Design review of the part built by this model. Coordinates are the model's own, in mm. Round coordinates to 2 decimals unless told otherwise and drop trailing zeros. Write each loop counter-clockwise with the first axis right and the second up, starting at its lowest first coordinate (ties: lowest second). Pieces come first, ordered by that corner, then holes. Notation, with made-up numbers: (64, 45) -> (84, 45) arc R17 ccw to (84, 49) -> close; hole circle Ø4 at (36, 32.5). An arc over 180 degrees is marked (long way). One line per question, with ' | ' between items. Start each with the question number.
1) Consider section A-A (x = 12). Give the boundary of the cut face in (y, z), then the cut area to 3 significant figures.
2) Consider section C-C (y = -17.5). Give the boundary of the cut face in (x, z), then the cut area to 3 significant figures.
3) Consider section B-B (y = -11.5). Give the boundary of the cut face in (x, z).
4) For probe 1 along Y at (x, z) = (12, 1.45); probe 2 along X at (y, z) = (-31, 5.1); probe 3 along X at (y, z) = (-5.5, 4.85), list the stretches that pass through material, from the lowest coordinate up.
5) Mouldability with a two-part tool opening along Y and no side actions: class faces 1 (the flat face through (90, -18, 3)), 2 (the cylindrical face through (10.4, -22.3, 3)), 3 (the flat face through (46, 0, 3)) as +Y half, -Y half, draft (parallel to the pull), parting line (faces both ways), or undercut.
6) Consider section D-D (z = 1). Count the separate pieces of the cut face and the enclosed holes in it, then the cut area to 3 significant figures.
Autodesk Inventor part; units mm, degrees
ref_plane "YZ Plane" through (0, 0, 0) normal (1, 0, 0) x (0, 1, 0)
ref_plane "XZ Plane" through (0, 0, 0) normal (0, 1, 0) x (-1, 0, 0)
ref_plane "XY Plane" through (0, 0, 0) normal (0, 0, 1) x (1, 0, 0)
sketch "Esboço1" plane through (0, 0, 0) normal (0, 0, 1) x (1, 0, 0)
  line L0 (90, 0) -> (0, 0)
  line L1 (0, 0) -> (0, -35)
  line L2 (0, -35) -> (90, -35)
  line L3 (90, -35) -> (90, 0)
  circle A0 centre (65.3687, -7.1) radius 2.3
  circle A1 centre (23.3687, -29.5996) radius 2.3
  circle A2 centre (44.3687, -27.9) radius 2.3
  circle A3 centre (44.3687, -7.1) radius 2.3
  circle A4 centre (84.63, -17.5) radius 2.3
  circle A5 centre (5.3687, -17.5) radius 2.3
  circle A6 centre (65.3687, -27.9) radius 2.3
  circle A7 centre (23.3687, -5.4004) radius 2.3
  circle A8 centre (12, -11.5) radius 2
  circle A9 centre (12, -23.5) radius 2
  circle A10 centre (76, -17.5) radius 2
  circle A11 centre (6.2932, -5.4004) radius 2.3
  circle A12 centre (6.2932, -29.5996) radius 2.3
  circle A13 centre (82.6841, -5.4004) radius 2.3
  circle A14 centre (82.6768, -29.5996) radius 2.3
extrude "Extrusão1" add sketch "Esboço1" along normal blind 6
properties part number "acrilico frontal" material "Acrílico, transparente"
From the geometry:
1) outline: (-35, 0) -> (-25.5, 0) -> (-25.5, 6) -> (-35, 6) -> close; (-21.5, 0) -> (-13.5, 0) -> (-13.5, 6) -> (-21.5, 6) -> close; (-9.5, 0) -> (0, 0) -> (0, 6) -> (-9.5, 6) -> close | area: 162 mm2
2) outline: (0, 0) -> (3.07, 0) -> (3.07, 6) -> (0, 6) -> close; (7.67, 0) -> (74, 0) -> (74, 6) -> (7.67, 6) -> close; (78, 0) -> (82.33, 0) -> (82.33, 6) -> (78, 6) -> close; (86.93, 0) -> (90, 0) -> (90, 6) -> (86.93, 6) -> close | area: 461 mm2
3) outline: (0, 0) -> (10, 0) -> (10, 6) -> (0, 6) -> close; (14, 0) -> (90, 0) -> (90, 6) -> (14, 6) -> close
4) probe 1: y = -35 to -25.5, -21.5 to -13.5, -9.5 to 0 | probe 2: x = 0 to 4.47, 8.12 to 21.54, 25.19 to 80.85, 84.5 to 90 | probe 3: x = 0 to 4, 8.59 to 21.07, 25.67 to 42.72, 46.02 to 63.72, 67.02 to 80.39, 84.98 to 90
5) face 1: draft | face 2: undercut | face 3: +Y half
6) separate pieces: 1 | enclosed holes: 15 | area: 2,910 mm2
